Part model, mm, in its own coordinate system. A direction names the side the tool comes from. Coordinates: 2 decimals unless noted, no trailing zeros. Loops run counter-clockwise (first coordinate to the right, second up) from the corner with the lowest first, then second, coordinate; pieces in that order, holes last. Notation, with made-up numbers: M 30.5,26.25 L 78.5,26.25 A27 ccw 78.5,56.25 Z; hole C 73.25,88 d9. An arc over 180 degrees is marked long. Answer as a JSON object with one key per item and string values. Group by question number.
1. Saw through at D-D on x = 5.5. Write the cut outline in (y, z).
2. Mould opens along Y. For faces 1 (the face through (15, 12.5, 12)), 2 (the face through (-2.14, 0.9, 3.04)), 3 (the face through (0, 8, 17)) say: released by +Y, released by -Y, zero draft, split by the parting line, or undercut.
3. Drill centre lines: L1, parallel to Y at x = 19, z = 2; L2, parallel to Y at x = -10, z = 9; L3, parallel to Z at x = -2, y = -5.5. Where is each one in solid material? Low to high.
4. Drop flat-ended pins along their axis: pin 1 Ø5.5 at (x, z) = (20, 9) entering from -Y; pin 2 Ø5 at (x, y) = (19, 0) entering from -Z; pin 3 Ø3.5 at (x, z) = (16.5, 11.5) entering from +Y; pin 4 Ø4 at (x, y) = (17, -16) entering from +Z. Give the stop position or say it passes through.
5. 3-axis set-ups, long thin cutter, end or side, ignore diameter. For faces 4 (the face through (-14, 0, 5)), 5 (the face through (4, 0, 6)), 6 (the face through (-0.353, 13.916, 11.577)), 7 (the face through (0, -7.5, 12)): which of +Z, -Z, +X, -X, +Y, -Y reach the whole face in a straight line?
6. Saw through at C-C on z = 15.5. Write the cut outline in (x, y).
7. Saw through at B-B on x = -5. Write the cut outline in (y, z).
8. Saw through at A-A on y = 0. Write the cut outline in (x, z).
from build123d import *

# Parameters (mm, degrees)
F0_W     = 54
F0_H     = 35
F1_DEPTH = 17
F2_W     = 13
F2_H     = 11
F3_DEPTH = 35
F5_DEPTH = 11
F6_W     = 30
F6_H     = 15
F6_R     = 3
F7_DEPTH = 11
F8_DEPTH = 25


with BuildPart() as f1:
    # F0 (on Top) → F1 (new body)
    with BuildSketch(Plane.XY):
        Rectangle(F0_W, F0_H)
    extrude(amount=F1_DEPTH)

    # F2 (on face) → F3 (cut)
    with BuildSketch(Plane.XZ.offset(17.5)):
        with Locations((-20.5, 5.5)):
            Rectangle(F2_W, F2_H)
    extrude(amount=-F3_DEPTH, mode=Mode.SUBTRACT)

    # F4 (on face) → F5 (cut)
    with BuildSketch(Plane.XY.offset(17)):
        with BuildLine():
            Line((4, -17.5), (27, -17.5))
            Line((27, -17.5), (27, -12.5))
            Line((27, -12.5), (4, -12.5))
            ThreePointArc((4, -12.5), (-0.3011626335, -13.8783723131), (-3, -17.5))
            Line((-3, -17.5), (4, -17.5))
        make_face()
        with BuildLine():
            ThreePointArc((-3, 17.5), (-0.3011626335, 13.8783723131), (4, 12.5))
            Line((4, 12.5), (27, 12.5))
            Line((27, 12.5), (27, 17.5))
            Line((27, 17.5), (4, 17.5))
            Line((4, 17.5), (-3, 17.5))
        make_face()
    extrude(amount=-F5_DEPTH, mode=Mode.SUBTRACT)

    # F6 (on face) → F7 (cut)
    with BuildSketch(Plane.XY.offset(17)):
        with Locations((0.5, 0)):
            Rectangle(F6_W, F6_H)
        with Locations((-5, 0)):
            Circle(F6_R, mode=Mode.SUBTRACT)
        with BuildLine():
            Line((15.5, 7.5), (15.5, -7.5))
            ThreePointArc((15.5, -7.5), (23, 0), (15.5, 7.5))
        make_face()
        with Locations((19, 0)):
            Circle(F6_R, mode=Mode.SUBTRACT)
        with BuildLine():
            ThreePointArc((-14.5, 7.5), (-22, 0), (-14.5, -7.5))
            Line((-14.5, -7.5), (-14.5, 7.5))
        make_face()
    extrude(amount=-F7_DEPTH, mode=Mode.SUBTRACT)

    # F8 (cut): faces of the model
    f8_faces = [f1.faces().sort_by_distance(p)[0] for p in [
        (-5, 0, 17),
        (19, 0, 17),
    ]]
    extrude(f8_faces, amount=-F8_DEPTH, mode=Mode.SUBTRACT)


solid = f1.part
Outcome:
{
 "1": {"outline": "M -17.5,0 L 17.5,0 L 17.5,6 L 12.5,6 L 12.5,17 L 7.5,17 L 7.5,6 L -7.5,6 L -7.5,17 L -12.5,17 L -12.5,6 L -17.5,6 Z"},
 "2": {"face 1": "released by +Y", "face 2": "undercut", "face 3": "zero draft"},
 "3": {"L1": "y = -17.5 to -3, 3 to 17.5", "L2": "y = -17.5 to -7.5, 7.5 to 17.5", "L3": "z = 0 to 6"},
 "4": {"pin 1": "stops at y = -12.5", "pin 2": "passes through", "pin 3": "stops at y = 12.5", "pin 4": "stops at z = 6"},
 "5": {"face 4": "-Z, -X, +Y, -Y", "face 5": "+Z, -X", "face 6": "+Z, +X, +Y", "face 7": "+Z"},
 "6": {"outline": "M -27,-17.5 L -3,-17.5 A7.4 cw 4,-12.5 L 27,-12.5 L 27,12.5 L 4,12.5 A7.4 cw -3,17.5 L -27,17.5 Z; hole M -14.5,-7.5 L 15.5,-7.5 A7.5 ccw 15.5,7.5 L -14.5,7.5 A7.5 ccw Z"},
 "7": {"outline": "M -17.5,0 L -3,0 L -3,6 L -7.5,6 L -7.5,17 L -17.5,17 Z; M 3,0 L 17.5,0 L 17.5,17 L 7.5,17 L 7.5,6 L 3,6 Z"},
 "8": {"outline": "M -27,11 L -22,11 L -22,17 L -27,17 Z; M -14,0 L -8,0 L -8,6 L -14,6 Z; M -2,0 L 16,0 L 16,6 L -2,6 Z; M 22,0 L 27,0 L 27,17 L 23,17 L 23,6 L 22,6 Z"}
}
